from build123d import *

# Parameters (mm, degrees)
SKETCH2_W           = 10
SKETCH2_H           = 5.5
BOSS_EXTRUDE1_DEPTH = 2.75
SKETCH3_R           = 2.25
CUT_EXTRUDE1_DEPTH  = 5
SKETCH4_W           = 2
SKETCH4_H           = 4.8
BOSS_EXTRUDE2_DEPTH = 4


with BuildPart() as part:
    # Sketch2 → Boss-Extrude1 (new, symmetric)
    with BuildSketch(Plane.XY):
        Rectangle(SKETCH2_W, SKETCH2_H)
    extrude(amount=BOSS_EXTRUDE1_DEPTH, both=True)

    # Sketch3 → Cut-Extrude1 (cut)
    with BuildSketch(Plane(origin=(5, 0, 0), x_dir=(0, 0, -1), z_dir=(1, 0, 0))):
        with Locations(Location((0, 0, 0), (0, 0, 90))):
            Circle(SKETCH3_R)
    extrude(amount=-CUT_EXTRUDE1_DEPTH, mode=Mode.SUBTRACT)

    # Sketch4 → Boss-Extrude2 (add)
    with BuildSketch(Plane(origin=(0, 2.75, 0), x_dir=(1, 0, 0), z_dir=(0, 1, 0))):
        with Locations((4, 0)):
            Rectangle(SKETCH4_W, SKETCH4_H)
    extrude(amount=BOSS_EXTRUDE2_DEPTH)


solid = part.part
Input: part model. Units: mm. Frame: model coordinates. A direction names the side the tool comes from. Give positions to 0.01 mm unless a question says otherwise; leave off trailing zeros. Write each loop counter-clockwise with the first axis right and the second up, starting at its lowest first coordinate (ties: lowest second). Pieces come first, ordered by that corner, then holes. Notation, with made-up numbers: M 78.25,27 L 91.25,27 A25 ccw 91.25,56 Z; hole C 1.5,68.5 d3. An arc over 180 degrees is marked long. Write item = value, one per line. Start each with the question number.
1) Reachability of faces 4 (the flat face through (4, 5, 2.4)), 5 (the cylindrical face through (2.535, 2.146, 0.676)), 6 (the flat face through (4, 5, -2.4)) from +Z, -Z, +X, -X, +Y, -Y: full face, straight path, thin tool, end or side. Return the list, or none.
2) Cut plane A-A on z = 0. Return the cut outline in (x, y).
3) Cut plane D-D on x = 2.25. Return the cut outline in (y, z), then the cut area to 3 significant figures.
4) Cut plane C-C on y = 0. Return the cut outline in (x, z).
5) Draft query along Y for faces 1 (the flat face through (4, 6.75, 0)), 2 (the flat face through (0, 0, 0)), 3 (the flat face through (0, 0, -2.75)). Return one class per face: +Y half, -Y half, draft (parallel to the pull), parting line (faces both ways), or undercut.
6) Cut plane B-B on x = 4.25. Return the cut outline in (y, z).
7) Material intervals for line 1 along Z through (x, y) = (1.8, 0); line 2 along X through (y, z) = (4.5, 1.7); line 3 along X through (y, z) = (-0.25, 2.2), sorted ascending. Write a range as [from, to].
8) First-contact query: pin 1 Ø3 at (y, z) = (6, -2) entering from -X; pin 2 Ø1 at (x, y) = (4, 4) entering from -Z; pin 3 Ø1.6 at (x, z) = (-2, -1) entering from +Y. Flat tips, straight axial feed; report the tip coordinate or a pass-through.
Solved:
q1.face_4 = +Z, +X, -X, +Y
q1.face_5 = +X
q1.face_6 = -Z, +X, -X, +Y
q2.outline = M -5,-2.75 L 5,-2.75 L 5,-2.25 L 0,-2.25 L 0,2.25 L 5,2.25 L 5,6.75 L 3,6.75 L 3,2.75 L -5,2.75 Z
q3.outline = M -2.75,-2.75 L 2.75,-2.75 L 2.75,2.75 L -2.75,2.75 Z; hole C 0,0 d4.5
q3.area = 14.3 mm2
q4.outline = M -5,-2.75 L 5,-2.75 L 5,-2.25 L 0,-2.25 L 0,2.25 L 5,2.25 L 5,2.75 L -5,2.75 Z
q5.face_1 = +Y half
q5.face_2 = undercut
q5.face_3 = draft
q6.outline = M -2.75,-2.75 L 2.75,-2.75 L 2.75,-2.4 L 6.75,-2.4 L 6.75,2.4 L 2.75,2.4 L 2.75,2.75 L -2.75,2.75 Z; hole C 0,0 d4.5
q7.line_1 = [-2.75, -2.25], [2.25, 2.75]
q7.line_2 = [3, 5]
q7.line_3 = [-5, 0]
q8.pin_1 = 3
q8.pin_2 = -2.4
q8.pin_3 = 2.75
